```python
from build123d import *

# Parameters (mm, degrees)
SKETCH1_R           = 12.5
BOSS_EXTRUDE1_DEPTH = 4
SKETCH2_R           = 7
BOSS_EXTRUDE2_DEPTH = 30
CHAMFER1_SIZE       = 2


with BuildPart() as part:
    # Sketch1 → Boss-Extrude1 (new body)
    with BuildSketch(Plane.XY):
        Circle(SKETCH1_R)
    extrude(amount=BOSS_EXTRUDE1_DEPTH)

    # Sketch2 → Boss-Extrude2 (add)
    with BuildSketch(Plane.XY.offset(4)):
        Circle(SKETCH2_R)
    extrude(amount=BOSS_EXTRUDE2_DEPTH)

    # Chamfer1
    chamfer1_edges = [part.edges().sort_by_distance(p)[0] for p in [
        (-12.5, 0, 0),
    ]]
    chamfer(chamfer1_edges, length=CHAMFER1_SIZE)


solid = part.part
```
The listing builds one solid part. Answer for the finished solid, in the listing's coordinates (mm). A direction names the side the tool comes from. Coordinates: 2 decimals unless noted, no trailing zeros. Write each loop counter-clockwise with the first axis right and the second up, starting at its lowest first coordinate (ties: lowest second). Pieces come first, ordered by that corner, then holes. Notation, with made-up numbers: (34, -13.5) - (44, -13.5) arc R27 cw to (44, 8.5) - close; hole circle Ø7 at (16, -2). An arc over 180 degrees is marked (long way). One line per item, written item: value.
1) Find section C-C (z = 16.5). Give the vertices of the cut face in (x, y).
Geometry check:
outline: circle Ø14 at (0, 0)
2) A tool of negligible diameter and unlimited length cuts with its end or side. For faces 1 (the flat face through (0, 0, 0)), 2 (the flat face through (5.4, -5.4, 4)), from which of +Z, -Z, +X, -X, +Y, -Y can it reach the whole face along a straight path? Write none if from no direction.
Geometry check:
face 1: -Z, +X, -X, +Y, -Y
face 2: +Z
3) Consider line 1 along Z through (x, y) = (-9, 5.25); line 2 along Y through (x, z) = (-2, 15); line 3 along Z through (x, y) = (-10.25, -7). Determine where each line is inside the solid, lowest interval first. Write a range as from..to.
Geometry check:
line 1: z = 0..4
line 2: y = -6.71..6.71
line 3: z = 1.91..4
4) Find section A-A (y = 0). Give the vertices of the cut face in (x, z).
Geometry check:
outline: (-12.5, 2) - (-10.5, 0) - (10.5, 0) - (12.5, 2) - (12.5, 4) - (7, 4) - (7, 34) - (-7, 34) - (-7, 4) - (-12.5, 4) - close
5) Each of these flat-tipped pins is pushed along its axis until it touches: pin 1 Ø10 at (x, y) = (3.5, 8.5) entering from +Z; pin 2 Ø5 at (y, z) = (-4.5, 24) entering from +X; pin 3 Ø10 at (y, z) = (1, 26) entering from +X; pin 4 Ø3 at (y, z) = (-1, 7) entering from -X. Where does it stop, or does it pass through?
Geometry check:
pin 1: stops at z = 34
pin 2: stops at x = 6.71
pin 3: stops at x = 7
pin 4: stops at x = -7
